Job drawing, mm, ordinate dimensions from the low corner. One solid piece. A direction names the side the tool comes from. Round coordinates to 2 decimals unless told otherwise and drop trailing zeros. Write each loop counter-clockwise with the first axis right and the second up, starting at its lowest first coordinate (ties: lowest second). Pieces come first, ordered by that corner, then holes. Notation, with made-up numbers: M 49,-23 L 100,-23 A19 cw 100,-12 Z; hole C -21.5,83.5 d3. An arc over 180 degrees is marked long. Answer as a JSON object with one key per item and string values. Group by question number.
1. Drop flat-ended pins along their axis: pin 1 (12 mm diameter, centred on x = 402, z = 278, fed in from -Y); pin 2 (3 mm diameter, centred on x = 497, z = 290.5, fed in from +Y); pin 3 (5 mm diameter, centred on x = 672.5, y = 33, fed in from +Z); pin 4 (12 mm diameter, centred on x = 827, y = 80.5, fed in from +Z). Give the stop position or say it passes through.
2. Band-saw the part on A-A, the plane z = 99. Write the cut outline in (x, y), plus the area to 3 significant figures.
3. Drill centre lines: line 1 (X direction, y = 57, z = 211); line 2 (Y direction, x = 586, z = 557); line 3 (Z direction, x = 822, y = 97). Where is each one in solid material? Low to high. Write a range as from..to.
4. Which spindle directions (+Z, -Z, +X, -X, +Y, -Y) get a long thin tool onto all of the face, cutting with end or side? Do the marked faces 3, 4 and 5. Say none if no direction does.
5. Band-saw the part on C-C, the plane y = 27. Write the cut outline in (x, z), plus the area to 3 significant figures.
6. Two-plate mould, pull along Z, no slides. Class the marked faces 1 and 2: +Z half, -Z half, draft (parallel to the pull), parting line (faces both ways), or undercut.
7. Band-saw the part on B-B, the plane x = 938. Write the cut outline in (y, z).
8. Band-saw the part on D-D, the plane z = 533.5. Write the cut outline in (x, y), plus the area to 3 significant figures.
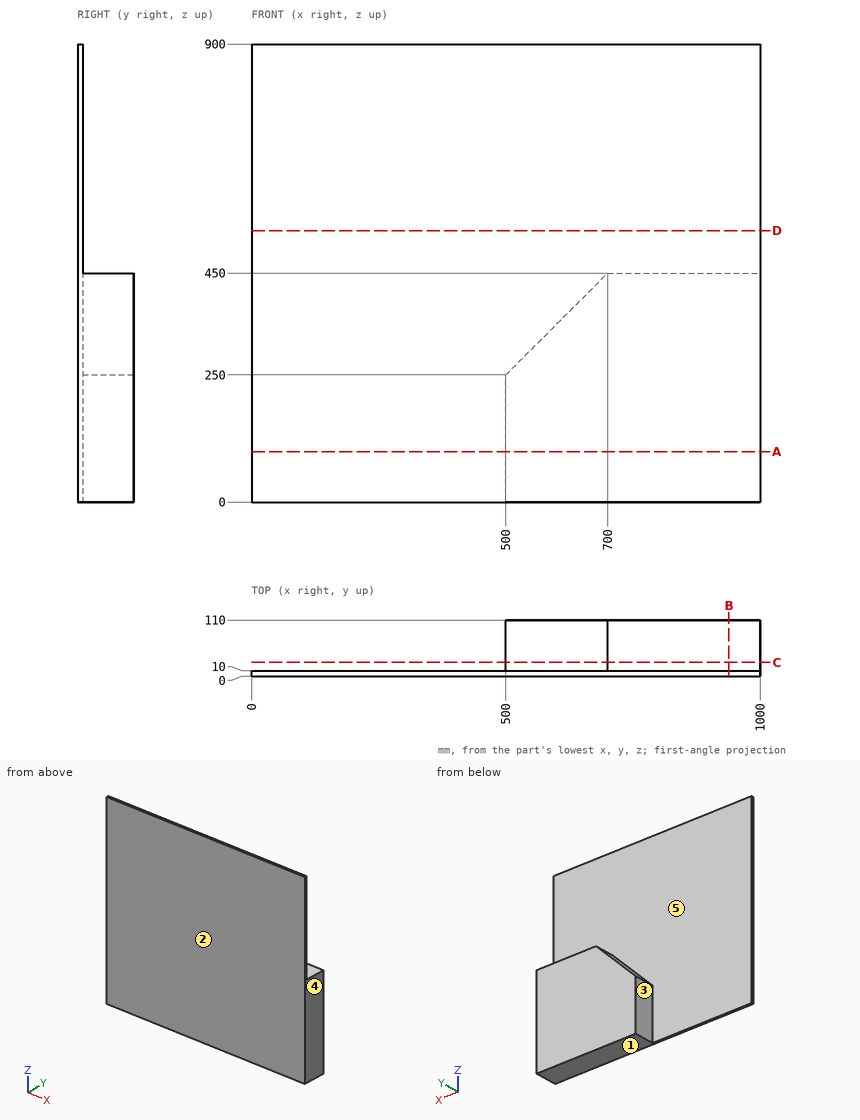
Worked answers:
{
 "1": {"pin 1": "stops at y = 0", "pin 2": "stops at y = 10", "pin 3": "stops at z = 425", "pin 4": "stops at z = 450"},
 "2": {"outline": "M 0,0 L 1000,0 L 1000,110 L 500,110 L 500,10 L 0,10 Z", "area": "60,000 mm^2"},
 "3": {"line 1": "x = 500..1000", "line 2": "y = 0..10", "line 3": "z = 0..450"},
 "4": {"face 3": "+Z, -Z, -X, +Y", "face 4": "+Z, -Z, +X, +Y, -Y", "face 5": "+Z, -X, +Y"},
 "5": {"outline": "M 500,0 L 1000,0 L 1000,450 L 700,450 L 500,250 Z", "area": "205,000 mm^2"},
 "6": {"face 1": "-Z half", "face 2": "draft"},
 "7": {"outline": "M 0,0 L 110,0 L 110,450 L 10,450 L 10,900 L 0,900 Z"},
 "8": {"outline": "M 0,0 L 1000,0 L 1000,10 L 0,10 Z", "area": "10,000 mm^2"}
}
